Can you work these out from the model? Positions are in its coordinate system, mm. A direction names the side the tool comes from. Round coordinates to 2 decimals unless told otherwise and drop trailing zeros. Loops run counter-clockwise (first coordinate to the right, second up) from the corner with the lowest first, then second, coordinate; pieces in that order, holes last.
(1) I want a section at A-A on x = -22. Write out the boundary of the cut face in (y, z).
(2) I want a section at B-B on y = 15. Write out the boundary of the cut face in (x, z), plus the area to 3 significant figures.
(3) I want a section at C-C on z = 6.5. Write out the boundary of the cut face in (x, y).
(4) Which directions (+Z, -Z, +X, -X, +Y, -Y) give clear straight access to the entire face, cutting with the end or side of a thin tool? Please do faces 1 (the face through (-1, 60, 5)), 2 (the face through (50, 2, 10)).
(5) Thinking about a two-plate mould opening in Y: for faces 3 (the face through (37.5, -1, 5)), 4 (the face through (127.5, -2, 4)), 5 (the face through (-2, -170, 4)), 6 (the face through (-37.5, -1, 5)), which applies, released by +Y, released by -Y, zero draft, split by the parting line, or undercut?
(6) If I drill on line 1 along Y through (x, z) = (20, 4.25); line 2 along X through (y, z) = (59, 8); line 3 along X through (y, z) = (-50.5, 9.5), over which ranges is the centre line in solid material (lowest first)?
(7) Will these pins go through, and if not, where does the flat tip stop? pin 1 Ø0.5 at (y, z) = (-71, 9.5) entering from +X; pin 2 Ø0.5 at (y, z) = (-62, 9.5) entering from -X.
from build123d import *

# Parameters (mm, degrees)
ESQUISSE1_W             = 255
ESQUISSE1_H             = 340
BOSS_EXTRU_1_DEPTH      = 10
ESQUISSE2_W             = 255
ESQUISSE2_H             = 340
ESQUISSE2_W_2           = 233
ESQUISSE2_H_2           = 318
ENL_V_MAT_EXTRU_1_DEPTH = 1
SKETCH1_W               = 75
SKETCH1_H               = 120
CUT_EXTRUDE1_DEPTH      = 20


with BuildPart() as part:
    # Esquisse1 → Boss.-Extru.1 (new body)
    with BuildSketch(Plane.XY):
        Rectangle(ESQUISSE1_W, ESQUISSE1_H)
    extrude(amount=BOSS_EXTRU_1_DEPTH)

    # Esquisse2 → Enlèv. mat.-Extru.1 (cut)
    with BuildSketch(Plane.XY.offset(10)):
        Rectangle(ESQUISSE2_W, ESQUISSE2_H)
        Rectangle(ESQUISSE2_W_2, ESQUISSE2_H_2, mode=Mode.SUBTRACT)
    extrude(amount=-ENL_V_MAT_EXTRU_1_DEPTH, mode=Mode.SUBTRACT)

    # Sketch1 → Cut-Extrude1 (cut)
    with BuildSketch(Plane.XY.offset(10)):
        Rectangle(SKETCH1_W, SKETCH1_H)
    extrude(amount=-CUT_EXTRUDE1_DEPTH, mode=Mode.SUBTRACT)


solid = part.part
Filled sheet:
1. outline: (-170, 0) - (-60, 0) - (-60, 10) - (-159, 10) - (-159, 9) - (-170, 9) - close; (60, 0) - (170, 0) - (170, 9) - (159, 9) - (159, 10) - (60, 10) - close
2. outline: (-127.5, 0) - (-37.5, 0) - (-37.5, 10) - (-116.5, 10) - (-116.5, 9) - (-127.5, 9) - close; (37.5, 0) - (127.5, 0) - (127.5, 9) - (116.5, 9) - (116.5, 10) - (37.5, 10) - close
2. area: 1,780 mm2
3. outline: (-127.5, -170) - (127.5, -170) - (127.5, 170) - (-127.5, 170) - close; hole (-37.5, -60) - (37.5, -60) - (37.5, 60) - (-37.5, 60) - close
4. face 1: +Z, -Z
4. face 2: +Z, +X, -X, +Y, -Y
5. face 3: undercut
5. face 4: zero draft
5. face 5: released by -Y
5. face 6: undercut
6. line 1: y = -170 to -60, 60 to 170
6. line 2: x = -127.5 to -37.5, 37.5 to 127.5
6. line 3: x = -116.5 to -37.5, 37.5 to 116.5
7. pin 1: stops at x = 116.5
7. pin 2: stops at x = -116.5
